Here's the drawing with two shaded views (mm, measured from the low corner). I have some questions. A direction names the side the tool comes from. Coordinates: 2 decimals unless noted, no trailing zeros. Order: outer loops, then holes, each group sorted by start corner. A loop starts at its lowest first (then second) coordinate and runs counter-clockwise, first axis right, second up. Notation, with made-up numbers: (80, 21) - (95, 21) arc R15 cw to (95, 40) - close; hole circle Ø5 at (30, 55.5). An arc over 180 degrees is marked (long way). Answer as a JSON object with one key per item and string values. Group by question number.
(1) Imagine slicing it at D-D, the plane z = 40. Write out the boundary of the cut face in (x, y), and give its area (3 significant figures).
(2) Please list where these lines run through material, in increasing order: probe 1 along Y at (x, z) = (40, 15.5); probe 2 along Y at (x, z) = (80, 6); probe 3 along Z at (x, y) = (53.5, 27).
(3) Imagine slicing it at B-B, the plane y = 50. Write out the boundary of the cut face in (x, z).
(4) Which directions (+Z, -Z, +X, -X, +Y, -Y) give clear straight access to the entire face, cutting with the end or side of a thin tool? Please do the marked faces 1, 2 and 3.
(5) We'd pull the mould along Y, two halves only. Please class the marked faces 4, 5 and 6: pulls with the +Y half, pulls with the -Y half, needs draft (parallel to the pull), parting line crosses it, or undercut.
(6) Imagine slicing it at C-C, the plane z = 12. Write out the boundary of the cut face in (x, y), and give its area (3 significant figures).
(7) Imagine slicing it at A-A, the plane x = 80. Write out the boundary of the cut face in (y, z), and give its area (3 significant figures).
(8) Will these pins go through, and if not, where does the flat tip stop? P1, Ø1.5, axis at y = 37.5, z = 21, coming from the -X side; P2, Ø8, axis at x = 71.5, y = 30.5, coming from the +Z side; P3, Ø8, axis at y = 26, z = 42.5, coming from the -X side; P4, Ø6, axis at x = 42.5, y = 6.5, coming from the -Z side.
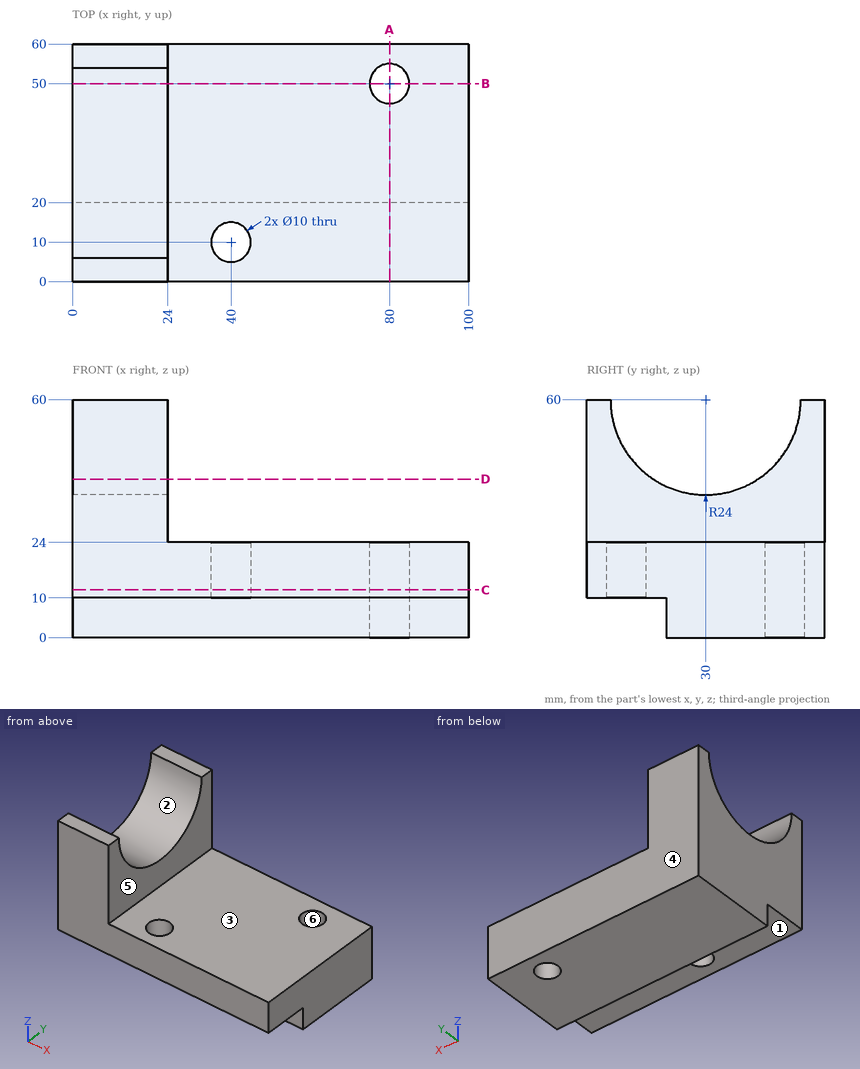
Result set:
{
 "1": {"outline": "(0, 0) - (24, 0) - (24, 16.73) - (0, 16.73) - close; (0, 43.27) - (24, 43.27) - (24, 60) - (0, 60) - close", "area": "803 mm^2"},
 "2": {"probe 1": "y = 0 to 5, 15 to 60", "probe 2": "y = 20 to 45, 55 to 60", "probe 3": "z = 0 to 24"},
 "3": {"outline": "(0, 0) - (75, 0) - (75, 24) - (24, 24) - (24, 46.73) - (0, 46.73) - close; (85, 0) - (100, 0) - (100, 24) - (85, 24) - close"},
 "4": {"face 1": "-Z, +X, -X, -Y", "face 2": "+Z, +X, -X", "face 3": "+Z, +X, +Y, -Y"},
 "5": {"face 4": "pulls with the +Y half", "face 5": "needs draft", "face 6": "undercut"},
 "6": {"outline": "(0, 0) - (100, 0) - (100, 60) - (0, 60) - close; hole circle Ø10 at (40, 10); hole circle Ø10 at (80, 50)", "area": "5,840 mm^2"},
 "7": {"outline": "(0, 10) - (20, 10) - (20, 0) - (45, 0) - (45, 24) - (0, 24) - close; (55, 0) - (60, 0) - (60, 24) - (55, 24) - close", "area": "1,000 mm^2"},
 "8": {"P1": "stops at x = 0", "P2": "stops at z = 24", "P3": "passes through", "P4": "stops at z = 10"}
}
